Verification items for the finished model (mm, model axes). A direction names the side the tool comes from. Coordinates: 2 decimals unless noted, no trailing zeros. Order: outer loops, then holes, each group sorted by start corner. A loop starts at its lowest first (then second) coordinate and runs counter-clockwise, first axis right, second up. Notation, with made-up numbers: M -15,20 L 19,20 A20 cw 19,39 Z; hole C -11,28.25 d4. An arc over 180 degrees is marked long. Return JSON: item names as keys, results as strings.
```python
from build123d import *

# Parameters (mm, degrees)
SKETCH1_R   = 1.25
BODY_DEPTH  = 5
END_DEPTH   = 1
SKETCH3_R   = 1
SCREW_DEPTH = 5


with BuildPart() as part:
    # Sketch1 → Body (new body)
    with BuildSketch(Plane(origin=(0, 0, 0), x_dir=(1, 0, 0), z_dir=(0, 1, 0))):
        Polygon((0, 2.5), (-2.165063509, 1.25), (-2.165063509, -1.25), (0, -2.5), (2.165063509, -1.25), (2.165063509, 1.25), align=None)
        with Locations(Location((0, 0, 0), (0, 0, 270))):
            Circle(SKETCH1_R, mode=Mode.SUBTRACT)
    extrude(amount=BODY_DEPTH)

    # Sketch2 → End (add)
    with BuildSketch(Plane.XZ):
        Polygon((0, -2.5), (2.165063509, -1.25), (2.165063509, 1.25), (0, 2.5), (-2.165063509, 1.25), (-2.165063509, -1.25), align=None)
    extrude(amount=END_DEPTH)

    # Sketch3 → Screw (add)
    with BuildSketch(Plane.XZ.offset(1)):
        with Locations(Location((0, 0, 0), (0, 0, 270))):
            Circle(SKETCH3_R)
    extrude(amount=SCREW_DEPTH)


solid = part.part
```
Q1. Cross-section at D-D, the plane y = -2. Record the boundary of the cut face in (x, z), and give its area (3 significant figures).
Values:
{"outline": "C 0,0 d2", "area": "3.14 mm^2"}
Q2. Go/stop test with a flat-tipped pin: pin 1 (1.5 mm diameter, centred on x = -1, y = -3, fed in from -Z). Record where the tip stops, or that it passes through.
Values:
{"pin 1": "z = -0.97"}
Q3. Cross-section at C-C, the plane x = 0.5. Record the boundary of the cut face in (y, z), and give its area (3 significant figures).
Values:
{"outline": "M -6,-0.87 L -1,-0.87 L -1,-2.21 L 5,-2.21 L 5,-1.15 L 0,-1.15 L 0,1.15 L 5,1.15 L 5,2.21 L -1,2.21 L -1,0.87 L -6,0.87 Z", "area": "23.7 mm^2"}
Q4. Material ranges on line 1 along X through (y, z) = (2.3, 0); line 2 along Y through (x, z) = (-0.5, 0.75); line 3 along Y through (x, z) = (1.25, 0.95), recorded low to high.
Values:
{"line 1": "-2.17 to -1.25, 1.25 to 2.17", "line 2": "-6 to 0", "line 3": "-1 to 5"}
Q5. Cross-section at A-A, the plane y = 3. Record the boundary of the cut face in (x, z), and give its area (3 significant figures).
Values:
{"outline": "M -2.17,-1.25 L 0,-2.5 L 2.17,-1.25 L 2.17,1.25 L 0,2.5 L -2.17,1.25 Z; hole C 0,0 d2.5", "area": "11.3 mm^2"}
Q6. Tool access check on faces 1 (the face through (-2.165, 2, 0)), 2 (the face through (1, -1, -1)). Record the directions out of +Z, -Z, +X, -X, +Y, -Y that give a thin tool (end or side, any length) a straight path to the whole face; none if there is none.
Values:
{"face 1": "+Z, -Z, -X, +Y, -Y", "face 2": "-Y"}
Q7. Draft check along Z on faces 3 (the face through (0, 0, 0)), 4 (the face through (0, -6, 0)), 5 (the face through (-1.22, 2.46, -0.27)), 6 (the face through (-1, -3, 0)). Enter one of: pulls with the +Z half, pulls with the -Z half, needs draft (parallel to the pull), parting line crosses it, or undercut.
Values:
{"face 3": "undercut", "face 4": "needs draft", "face 5": "undercut", "face 6": "parting line crosses it"}
Q8. Cross-section at B-B, the plane z = 0. Record the boundary of the cut face in (x, y), and give its area (3 significant figures).
Values:
{"outline": "M -2.17,-1 L -1,-1 L -1,-6 L 1,-6 L 1,-1 L 2.17,-1 L 2.17,5 L 1.25,5 L 1.25,0 L -1.25,0 L -1.25,5 L -2.17,5 Z", "area": "23.5 mm^2"}
